```python
from build123d import *

# Parameters (mm, degrees)
F2_DEPTH  = 60
F3_DEPTH  = 60
F4_W      = 34.0656559074
F4_H      = 51.5325679444
F5_DEPTH  = 10
F6_W      = 51.5325679444
F6_H      = 15
F7_DEPTH  = 4
F8_W      = 51.9751724787
F8_H      = 31.6211068177
F9_DEPTH  = 15
F10_W     = 51.5005090274
F10_H     = 31.6510945126
F11_DEPTH = 6.8


with BuildPart() as f2:
    # F0 (on Front) → F2 (new body)
    with BuildSketch(Plane.XZ):
        Polygon((-17.8921578123, 20.3632246609), (-20.3399246612, 25.4550932741), (-55.7910754849, 6.9290061191), (-58.7328180983, -7.779703899), (-63.7328180983, -7.779703899), (-63.7328180983, -9.779703899), (-58.7328180983, -9.779703899), (-65.9274235368, -44.0322607756), (-62.9274235368, -44.0322607756), (-55.7910754849, -9.779703899), (-28.9112906903, -9.779703899), (-23.3467742801, -44.0322607756), (-20.3467742801, -44.0322607756), (-25.8926429036, -9.8944909401), (-20.8926429036, -9.8944909401), (-20.8926429036, -7.8944909401), (-25.8926429036, -7.8944909401), (-29.4905570809, 14.25258365), (-20.6433312194, 18.913763174), align=None)
    extrude(amount=F2_DEPTH)

    # F1 (on Front) → F3 (cut)
    with BuildSketch(Plane.XZ):
        with BuildLine():
            add(Edge.make_bspline(
                [(-32.0564545691, 8.4677422419), (-32.9182067785, 9.4601825496), (-34.6748450566, 11.4832219038), (-38.7271868794, 10.9055197371), (-52.1695896145, 5.7227527212), (-53.2214258813, 0.0155056606), (-54.7111549811, -4.8464931653), (-55.5241964757, -7.500000298)],
                knots=[0, 0, 0, 0, 0.1495745389, 0.3049001298, 0.5961488941, 0.7795923388, 1, 1, 1, 1], degree=3))
            Line((-55.5241964757, -7.500000298), (-29.6370983124, -7.500000298))
            Line((-29.6370983124, -7.500000298), (-32.0564545691, 8.4677422419))
        make_face()
    extrude(amount=F3_DEPTH, mode=Mode.SUBTRACT)

    # F4 (on face) → F5 (cut)
    with BuildSketch(Plane(origin=(-14.8119721989, 0, 28.3438945324), x_dir=(0.8862787706, 0, 0.4631521789), z_dir=(-0.4631521789, 0, 0.8862787706))):
        with Locations((-29.2044335556, -29.7510505188)):
            Rectangle(F4_W, F4_H)
    extrude(amount=-F5_DEPTH, mode=Mode.SUBTRACT)

    # F6 (on face) → F7 (cut)
    with BuildSketch(Plane(origin=(-54.9777654657, 0, 10.9955553723), x_dir=(0, -1, 0), z_dir=(-0.9805806679, 0, 0.1961161742))):
        with Locations((29.7510505188, -11.647082832)):
            Rectangle(F6_W, F6_H)
    extrude(amount=-F7_DEPTH, mode=Mode.SUBTRACT)

    # F8 (on face) → F9 (cut)
    with BuildSketch(Plane(origin=(-54.2836781091, 0, 11.4020581632), x_dir=(0, -1, 0), z_dir=(-0.9786444822, 0, 0.2055601554))):
        with Locations((30.0000028219, -40.8334270638)):
            Rectangle(F8_W, F8_H)
    extrude(amount=-F9_DEPTH, mode=Mode.SUBTRACT)

    # F10 (on face) → F11 (cut)
    with BuildSketch(Plane(origin=(-26.7929436535, 0, -4.3526611802), x_dir=(0, 1, 0), z_dir=(0.987059687, 0, 0.1603532795))):
        with Locations((-29.7626692336, -24.3742503009)):
            Rectangle(F10_W, F10_H)
    extrude(amount=-F11_DEPTH, mode=Mode.SUBTRACT)


solid = f2.part
```
Geometry: final body of the model. Coordinates: model frame, mm. A direction names the side the tool comes from. Give positions to 0.01 mm unless a question says otherwise; leave off trailing zeros. Order: outer loops, then holes, each group sorted by start corner. A loop starts at its lowest first (then second) coordinate and runs counter-clockwise, first axis right, second up. Notation, with made-up numbers: (69.25, -9.5) -> (128.25, -9.5) arc R22 cw to (128.25, 0.5) -> close; hole circle Ø5 at (-26, -36). An arc over 180 degrees is marked (long way). Write each question's results on one line, items separated by ' | '. Start each with the question number.
1) Section A-A (y = -48.5). Return loops of the section in (x, z) (1 decimal).
2) Section B-B (z = -37). Return loops of the section in (x, y).
3) Section C-C (x = -31). Return loops of the section in (y, z).
4) Section D-D (x = -38). Count the separate pieces of the cut face and the enclosed holes in it, then the cut area to 3 significant figures.
5) Line query: line 1 (Y direction, x = -34, z = 13); line 2 (Z direction, x = -42.5, y = -46); line 3 (Z direction, x = -21.5, y = -23). Output: solid intervals per line, ascending. Write a range as from..to.
6) Set-up query: faces 4 (the flat face through (-28.41, -29.86, -12.87)), 5 (the flat face through (-58.035, -29.636, -13.379)), 6 (the flat face through (-20.893, -30, -9)), 7 (the flat face through (-30.83, -29.58, 0.37)). Return all of +Z, -Z, +X, -X, +Y, -Y with unobstructed straight access to the full face (end or side cutting, diameter ignored); none if empty.
7) Draft query along Z for faces 1 (the flat face through (-61, -4.012, -29)), 2 (the flat face through (-59.38, -29.86, -12.87)), 3 (the flat face through (-61, -30, -7.78)). Return one class per face: pulls with the +Z half, pulls with the -Z half, needs draft (parallel to the pull), parting line crosses it, or undercut.
8) First-contact query: pin 1 (2.5 mm diameter, centred on x = -61, y = -40, fed in from +Z); pin 2 (1 mm diameter, centred on x = -39.5, y = -35.5, fed in from -Z); pin 3 (1.5 mm diameter, centred on x = -23, y = -43.5, fed in from -Z). Flat tips, straight axial feed; report the tip coordinate or a pass-through.
Calculated:
1) outline: (-63.7, -9.8) -> (-58.7, -9.8) -> (-59.4, -13.1) -> (-56.6, -13.7) -> (-55.8, -9.8) -> (-28.9, -9.8) -> (-28.3, -13.3) -> (-25.4, -12.8) -> (-25.9, -9.9) -> (-20.9, -9.9) -> (-20.9, -7.9) -> (-25.9, -7.9) -> (-28.8, 9.8) -> (-32, 8.1) -> (-29.6, -7.5) -> (-54.6, -7.5) -> (-54.8, -8.6) -> (-58.7, -7.8) -> (-63.7, -7.8) -> close; (-25.6, 22.7) -> (-23, 17.7) -> (-17.9, 20.4) -> (-20.3, 25.5) -> close
2) outline: (-64.45, -60) -> (-61.46, -60) -> (-61.46, -55.99) -> (-64.45, -55.99) -> close; (-64.45, -4.01) -> (-61.46, -4.01) -> (-61.46, 0) -> (-64.45, 0) -> close; (-24.49, -60) -> (-21.49, -60) -> (-21.49, -55.51) -> (-24.49, -55.51) -> close; (-24.49, -4.01) -> (-21.49, -4.01) -> (-21.49, 0) -> (-24.49, 0) -> close
3) outline: (-60, -9.78) -> (0, -9.78) -> (0, -7.5) -> (-60, -7.5) -> close; (-60, 1.5) -> (0, 1.5) -> (0, 19.88) -> (-3.98, 19.88) -> (-3.98, 8.6) -> (-55.52, 8.6) -> (-55.52, 19.88) -> (-60, 19.88) -> close
4) separate pieces: 3 | enclosed holes: 0 | area: 183 mm2
5) line 1: -60..-55.52, -3.98..0 | line 2: -9.78..-7.5 | line 3: -9.89..-7.89, 18.46..24.85
6) face 4: -Z, +Y, -Y | face 5: -Z, -X | face 6: +X, +Y, -Y | face 7: +Y, -Y
7) face 1: needs draft | face 2: undercut | face 3: pulls with the +Z half
8) pin 1: z = -7.78 | pin 2: z = -9.78 | pin 3: z = -9.89
